from build123d import *

# Parameters (mm, degrees)
SKETCH1_R           = 14
BOSS_EXTRUDE1_DEPTH = 50
CUT_EXTRUDE1_DEPTH  = 33
SKETCH3_R           = 9.5
CUT_EXTRUDE2_DEPTH  = 24.5
SKETCH5_R           = 1.5
CUT_EXTRUDE3_DEPTH  = 4.619168
CIRPATTERN1_COUNT   = 2
CIRPATTERN1_ANGLE   = 90


with BuildPart() as part:
    # Sketch1 → Boss-Extrude1 (new body)
    with BuildSketch(Plane(origin=(0, 0, 0), x_dir=(1, 0, 0), z_dir=(0, 1, 0))):
        with Locations(Location((0, 0, 0), (0, 0, 270))):  # turned: the seam where the file's is
            Circle(SKETCH1_R)
    extrude(amount=BOSS_EXTRUDE1_DEPTH)

    # Sketch2 → Cut-Extrude1 (cut)
    with BuildSketch(Plane(origin=(0, 0, 0), x_dir=(-1, 0, 0), z_dir=(0, -1, 0))):
        with BuildLine():
            Line((-2.397915762, -5.5), (2.397915762, -5.5))
            ThreePointArc((2.397915762, -5.5), (5.196152423, -3), (5.962097602, 0.673344034))
            Line((5.962097602, 0.673344034), (3.56418184, 4.826655966))
            ThreePointArc((3.56418184, 4.826655966), (0, 6), (-3.56418184, 4.826655966))
            Line((-3.56418184, 4.826655966), (-5.962097602, 0.673344034))
            ThreePointArc((-5.962097602, 0.673344034), (-5.196152423, -3), (-2.397915762, -5.5))
        make_face()
    extrude(amount=-CUT_EXTRUDE1_DEPTH, mode=Mode.SUBTRACT)

    # Sketch3 → Cut-Extrude2 (cut)
    with BuildSketch(Plane(origin=(0, 50, 0), x_dir=(1, 0, 0), z_dir=(0, 1, 0))):
        with Locations(Location((0, 0, 0), (0, 0, 270))):  # turned: the seam where the file's is
            Circle(SKETCH3_R)
    extrude(amount=-CUT_EXTRUDE2_DEPTH, mode=Mode.SUBTRACT)

    # Sketch5 → Cut-Extrude3 (cut)
    with BuildSketch(Plane(origin=(14, 50, 0), x_dir=(0, 0, -1), z_dir=(1, 0, 0))):
        with Locations((0, -2.3)):
            Circle(SKETCH5_R)
        with Locations((0, -18.3)):
            Circle(SKETCH5_R)
    cut_extrude3 = extrude(amount=-CUT_EXTRUDE3_DEPTH, mode=Mode.SUBTRACT)

    # CirPattern1: Cut-Extrude3 ×2 about axis
    cirpattern1_axis = Axis((0, 33, 0), (0, -1, 0))
    for i in range(1, CIRPATTERN1_COUNT):
        add(cut_extrude3.rotate(cirpattern1_axis, i * CIRPATTERN1_ANGLE / (CIRPATTERN1_COUNT - 1)), mode=Mode.SUBTRACT)


solid = part.part
Input: part model. Units: mm. Frame: model coordinates. A direction names the side the tool comes from. Round coordinates to 2 decimals unless told otherwise and drop trailing zeros. Order: outer loops, then holes, each group sorted by start corner. A loop starts at its lowest first (then second) coordinate and runs counter-clockwise, first axis right, second up. Notation, with made-up numbers: (28.25, 50.25) - (64.25, 50.25) arc R10 ccw to (64.25, 57.25) - close; hole circle Ø11 at (-12.5, 3). An arc over 180 degrees is marked (long way). Answer as a JSON object with one key per item and string values. Group by question number.
(1) Pin query (flat end, axial travel): P1, Ø1, axis at y = 28.5, z = 3, coming from the -X side (3 decimals); P2, Ø3, axis at y = 22, z = 6, coming from the -X side; P3, Ø3, axis at x = -10, y = 15.5, coming from the +Z side. Return the tip coordinate at first contact, or that it passes through.
(2) Material intervals for probe 1 along Y at (x, z) = (11.75, 0); probe 2 along X at (y, z) = (44.5, 0); probe 3 along X at (y, z) = (31.7, 10.4), sorted ascending. Write a range as from..to.
(3) Cut plane B-B (x = 0). Return loops of the section in (y, z).
(4) Cut plane C-C (y = 17). Return loops of the section in (x, z).
(5) Reachability of faces 5 (the face through (-4.1, 25.5, -4.4)), 6 (the face through (5.223, 12.572, 2.954)), 7 (the face through (11.723, 49.187, 0.195)) from +Z, -Z, +X, -X, +Y, -Y: full face, straight path, thin tool, end or side. Return the list, or none.
(6) Draft query along Y for faces 1 (the face through (-0.195, 49.187, 11.723)), 2 (the face through (11.723, 30.236, 0.325)), 3 (the face through (0, 13, -6)), 4 (the face through (-9.1, 50, -3.3)). Return one class per face: released by +Y, released by -Y, zero draft, split by the parting line, or undercut.
(7) Cut plane D-D (x = -4.25). Return loops of the section in (y, z), then the cut area to 3 significant figures.
(8) Cut plane A-A (z = 0). Return loops of the section in (x, y), then the cut area to 4 significant figures.
Here are the results:
{
 "1": {"P1": "stops at x = -13.775", "P2": "stops at x = -13.26", "P3": "stops at z = 11.12"},
 "2": {"probe 1": "y = 0..30.2, 33.2..46.2, 49.2..50", "probe 2": "x = -14..-9.5, 9.5..14", "probe 3": "x = -9.37..-1.5, 1.5..9.37"},
 "3": {"outline": "(0, -14) - (50, -14) - (50, -9.5) - (25.5, -9.5) - (25.5, -6) - (0, -6) - close; (0, 5.5) - (25.5, 5.5) - (25.5, 9.5) - (30.2, 9.5) - (30.2, 14) - (0, 14) - close; (33.2, 9.5) - (46.2, 9.5) - (46.2, 14) - (33.2, 14) - close; (49.2, 9.5) - (50, 9.5) - (50, 14) - (49.2, 14) - close"},
 "4": {"outline": "circle Ø28 at (0, 0); hole (-5.96, -0.67) - (-3.56, -4.83) arc R6 ccw to (3.56, -4.83) - (5.96, -0.67) arc R6 ccw to (2.4, 5.5) - (-2.4, 5.5) arc R6 ccw to start"},
 "5": {"face 5": "+Y", "face 6": "+Y, -Y", "face 7": "+X"},
 "6": {"face 1": "undercut", "face 2": "undercut", "face 3": "zero draft", "face 4": "released by +Y"},
 "7": {"outline": "(0, -13.34) - (50, -13.34) - (50, -8.5) - (25.5, -8.5) - (25.5, -3.64) - (0, -3.64) - close; (0, 4.24) - (25.5, 4.24) - (25.5, 8.5) - (50, 8.5) - (50, 13.34) - (0, 13.34) - close", "area": "717 mm^2"},
 "8": {"outline": "(-14, 0) - (-6, 0) - (-6, 25.5) - (-9.5, 25.5) - (-9.5, 50) - (-14, 50) - close; (6, 0) - (14, 0) - (14, 30.2) - (9.5, 30.2) - (9.5, 25.5) - (6, 25.5) - close; (9.5, 33.2) - (14, 33.2) - (14, 46.2) - (9.5, 46.2) - close; (9.5, 49.2) - (14, 49.2) - (14, 50) - (9.5, 50) - close", "area": "601.5 mm^2"}
}
